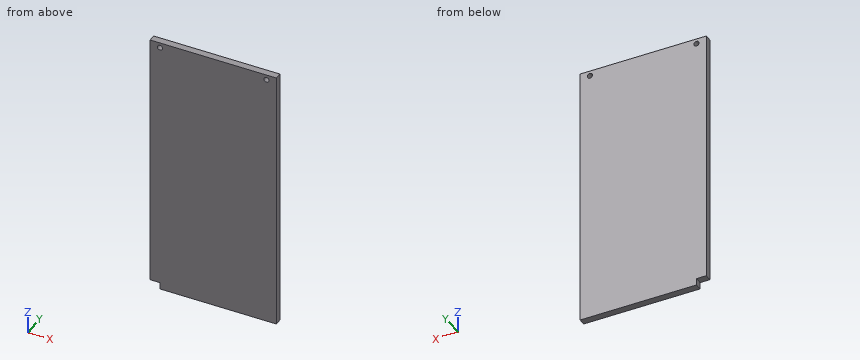
from build123d import *

# Parameters (mm, degrees)
SKETCH030_W     = 73.4
SKETCH030_H     = 156
PAD008_DEPTH    = 4
SKETCH031_R     = 1.5
POCKET014_DEPTH = 4
SKETCH032_W     = 14
SKETCH032_H     = 16
POCKET015_DEPTH = 5


with BuildPart() as part:
    # Sketch030 → Pad008 (new body)
    with BuildSketch(Plane.XZ):
        with Locations((45, 90)):
            Rectangle(SKETCH030_W, SKETCH030_H)
    extrude(amount=PAD008_DEPTH)

    # Sketch031 (on Face5 of Pad008) → Pocket014 (cut)
    with BuildSketch(Plane(origin=(0, 0, 0), x_dir=(1, 0, 0), z_dir=(0, 1, 0))):
        with Locations((14, -165)):
            Circle(SKETCH031_R)
        with Locations((76, -165)):
            Circle(SKETCH031_R)
    extrude(amount=-POCKET014_DEPTH, mode=Mode.SUBTRACT)

    # Sketch032 (on Face4 of Pocket014) → Pocket015 (cut)
    with BuildSketch(Plane(origin=(0, 0, 0), x_dir=(1, 0, 0), z_dir=(0, 1, 0))):
        with Locations((7, -8)):
            Rectangle(SKETCH032_W, SKETCH032_H)
    extrude(amount=-POCKET015_DEPTH, mode=Mode.SUBTRACT)


solid = part.part
For this review, take the finished solid that the model builds, in its own axes (mm). Coordinates: 2 decimals unless noted, no trailing zeros. Order: outer loops, then holes, each group sorted by start corner. A loop starts at its lowest first (then second) coordinate and runs counter-clockwise, first axis right, second up. Notation, with made-up numbers: (76.5, 40) -> (103.5, 40) arc R28 ccw to (103.5, 65) -> close; hole circle Ø1 at (70, 67.5). An arc over 180 degrees is marked (long way). Return JSON: item names as keys, results as strings.
1. For pin 1 Ø5 at (x, z) = (76, 165) entering from -Y; pin 2 Ø2 at (x, y) = (10, -1.5) entering from -Z, all flat-tipped, find the tip position at first contact; note any pin that passes through.
Answer block:
{"pin 1": "y = -4", "pin 2": "z = 16"}
2. For line 1 (X direction, y = -0.9, z = 165); line 2 (Z direction, x = 76, y = -1.35); line 3 (Z direction, x = 11, y = -2.8), list the stretches that pass through material, from the lowest coordinate up. Write a range as from..to.
Answer block:
{"line 1": "8.3..12.5, 15.5..74.5, 77.5..81.7", "line 2": "12..163.5, 166.5..168", "line 3": "16..168"}
3. We need section B-B on z = 165. Write out the cut boundary in (x, y), and give its area (3 significant figures).
Answer block:
{"outline": "(8.3, -4) -> (12.5, -4) -> (12.5, 0) -> (8.3, 0) -> close; (15.5, -4) -> (74.5, -4) -> (74.5, 0) -> (15.5, 0) -> close; (77.5, -4) -> (81.7, -4) -> (81.7, 0) -> (77.5, 0) -> close", "area": "270 mm²"}
4. We need section A-A on x = 76. Write out the cut boundary in (y, z).
Answer block:
{"outline": "(-4, 12) -> (0, 12) -> (0, 163.5) -> (-4, 163.5) -> close; (-4, 166.5) -> (0, 166.5) -> (0, 168) -> (-4, 168) -> close"}
